Input: dimensioned drawing with shaded views. Units: mm. Origin: part minimum x, y, z. A direction names the side the tool comes from. Give positions to 0.01 mm unless a question says otherwise; leave off trailing zeros. Write each loop counter-clockwise with the first axis right and the second up, starting at its lowest first coordinate (ties: lowest second). Pieces come first, ordered by that corner, then holes.
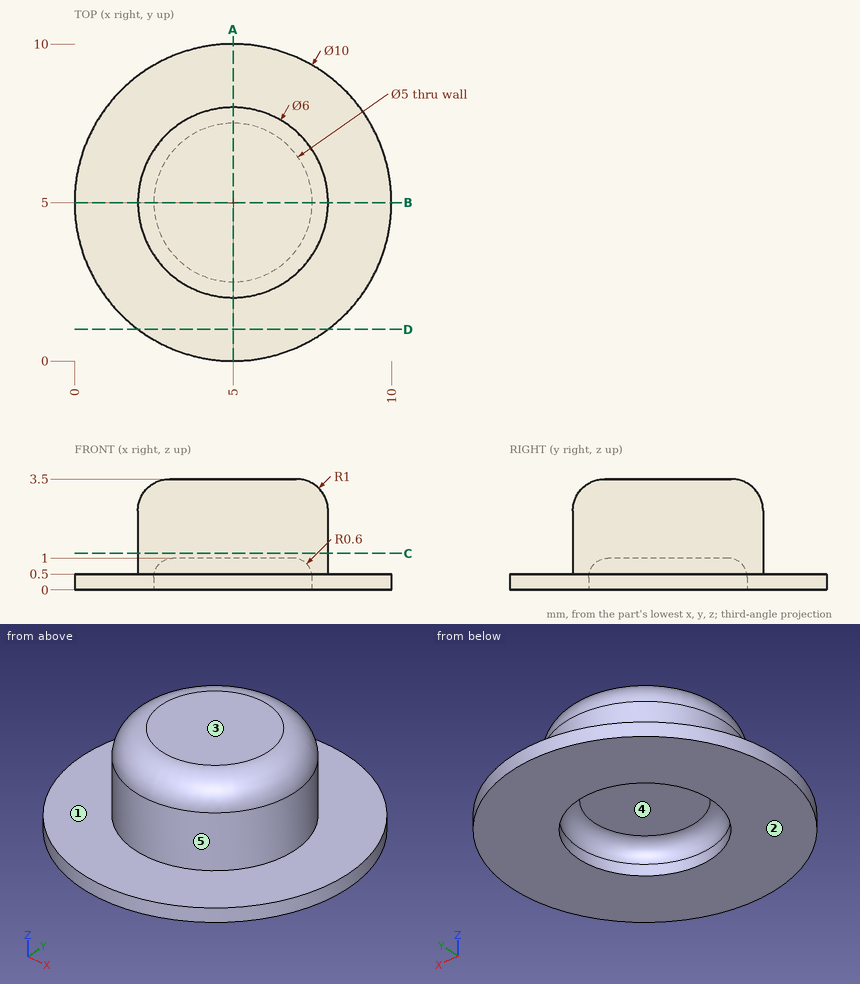
1. Line query: L1, parallel to Y at x = 5, z = 0.15; L2, parallel to Z at x = 1.75, y = 7; L3, parallel to Z at x = 6, y = 6. Output: solid intervals per line, ascending.
2. Mould query, pull axis X, two halves, no side actions, for the marked faces 3, 4 and 5. Classes: +X half, -X half, draft (parallel to the pull), parting line (faces both ways), or undercut.
3. Cut plane C-C, the plane z = 1.15. Return the cut outline in (x, y), then the cut area to 3 significant figures.
4. Cut plane A-A, the plane x = 5. Return the cut outline in (y, z), then the cut area to 3 significant figures.
5. Contact query for flat-ended pins moving along their axis: P1, Ø4, axis at x = 7.5, y = 9, coming from the +Z side; P2, Ø1, axis at x = 1.5, z = 0.5, coming from the +Y side; P3, Ø1.1, axis at x = 5.5, y = 5.5, coming from the -Z side. Output: stop coordinate, or through.
6. Access query for the marked faces 1 and 2. Directions: +Z, -Z, +X, -X, +Y, -Y. A direction counts if a zero-diameter tool reaches every point of the face in a straight line with its end or side. Return the directions, or none.
7. Cut plane D-D, the plane y = 1. Return the cut outline in (x, z), then the cut area to 3 significant figures.
Response values:
1. L1: y = 0 to 2.5, 7.5 to 10
1. L2: z = 0 to 0.5
1. L3: z = 1 to 3.5
2. face 3: draft
2. face 4: undercut
2. face 5: parting line
3. outline: circle Ø6 at (5, 5)
3. area: 28.3 mm2
4. outline: (0, 0) - (2.5, 0) - (2.5, 0.4) arc R0.6 cw to (3.1, 1) - (6.9, 1) arc R0.6 cw to (7.5, 0.4) - (7.5, 0) - (10, 0) - (10, 0.5) - (8, 0.5) - (8, 2.5) arc R1 ccw to (7, 3.5) - (3, 3.5) arc R1 ccw to (2, 2.5) - (2, 0.5) - (0, 0.5) - close
4. area: 17.7 mm2
5. P1: stops at z = 3.2
5. P2: stops at y = 9
5. P3: stops at z = 1
6. face 1: +Z
6. face 2: -Z, +X, -X, +Y, -Y
7. outline: (2, 0) - (8, 0) - (8, 0.5) - (2, 0.5) - close
7. area: 3.00 mm2
